Could you check a few things on this model? Use its own coordinates, in mm. Give positions to 0.01 mm unless a question says otherwise; leave off trailing zeros. Order: outer loops, then holes, each group sorted by start corner. A loop starts at its lowest first (then second) coordinate and runs counter-clockwise, first axis right, second up. Notation, with made-up numbers: (23.5, 23.25) -> (28.5, 23.25) arc R30 cw to (28.5, 57.25) -> close; hole circle Ø2 at (15, 69). An arc over 180 degrees is marked (long way). Use one line per item in the form item = value. Start each with the question number.
from build123d import *

# Parameters (mm, degrees)
F0_R     = 12.7
F1_DEPTH = 19.05
F2_R     = 2.54


with BuildPart() as f1:
    # F0 (on Front) → F1 (new body)
    with BuildSketch(Plane.XZ):
        Polygon((5.144296, -21.387057), (21.093883, -6.238438), (15.949587, 15.148619), (-5.144296, 21.387057), (-21.093883, 6.238438), (-15.949587, -15.148619), align=None)
        Circle(F0_R, mode=Mode.SUBTRACT)
    extrude(amount=F1_DEPTH)

    # F2
    f2_edges = [f1.edges().sort_by_distance(p)[0] for p in [
        (-5.402646, -19.05, -18.267838),
        (13.119089, -19.05, -13.812748),
        (18.521735, -19.05, 4.455091),
        (5.402646, -19.05, 18.267838),
        (-13.119089, -19.05, 13.812748),
        (-18.521735, -19.05, -4.455091),
        (-5.402646, 0, -18.267838),
        (-15.949587, -9.525, -15.148619),
        (-18.521735, 0, -4.455091),
        (-13.119089, 0, 13.812748),
        (5.402646, 0, 18.267838),
        (18.521735, 0, 4.455091),
        (13.119089, 0, -13.812748),
        (-21.093883, -9.525, 6.238438),
        (-5.144296, -9.525, 21.387057),
        (15.949587, -9.525, 15.148619),
        (21.093883, -9.525, -6.238438),
        (5.144296, -9.525, -21.387057),
    ]]
    fillet(f2_edges, radius=F2_R)


solid = f1.part
(1) I'm going to push flat-ended pins straight in: pin 1 Ø6 at (x, y) = (-1, -4.5) entering from -Z; pin 2 Ø4 at (y, z) = (-6, 14) entering from +X; pin 3 Ø1 at (x, z) = (-11.5, -16.5) entering from +Y. Where does each tip first touch, or does it pass through?
(2) Please list where these lines run through material, in increasing order: probe 1 along Z at (x, y) = (0, -11); probe 2 along Z at (x, y) = (9.5, -17.25); probe 3 along X at (y, z) = (-13, 10).
(3) We'd pull the mould along Z, two halves only. Please class faces 1 (the flat face through (4, -19.05, -12.3)), 2 (the cylindrical face through (15.68, -9.62, 14.86)), 3 (the cylindrical face through (-2.75, -9.39, -12.4)), 4 (the cylindrical face through (5.07, -9.62, -21)): pulls with the +Z half, pulls with the -Z half, needs draft (parallel to the pull), parting line crosses it, or undercut.
(4) Imagine slicing it at A-A (y = -8.75). Write out the boundary of the cut face in (x, z), plus the area to 3 significant figures.
Calculated:
q1.pin_1 = -20.46
q1.pin_2 = 16.71
q1.pin_3 = -1.07
q2.probe_1 = -19.87 to -12.7, 12.7 to 19.87
q2.probe_2 = -17.1 to -8.43, 8.43 to 16.94
q2.probe_3 = -17.13 to -7.83, 7.83 to 17.19
q3.face_1 = needs draft
q3.face_2 = pulls with the +Z half
q3.face_3 = undercut
q3.face_4 = pulls with the -Z half
q4.outline = (-20.75, 4.81) -> (-16.29, -13.72) arc R2.54 ccw to (-14.54, -15.56) -> (3.74, -20.97) arc R2.54 ccw to (6.21, -20.38) -> (20.03, -7.25) arc R2.54 ccw to (20.75, -4.81) -> (16.29, 13.72) arc R2.54 ccw to (14.54, 15.56) -> (-3.74, 20.97) arc R2.54 ccw to (-6.21, 20.38) -> (-20.03, 7.25) arc R2.54 ccw to start; hole circle Ø25.4 at (0, 0)
q4.area = 748 mm2
